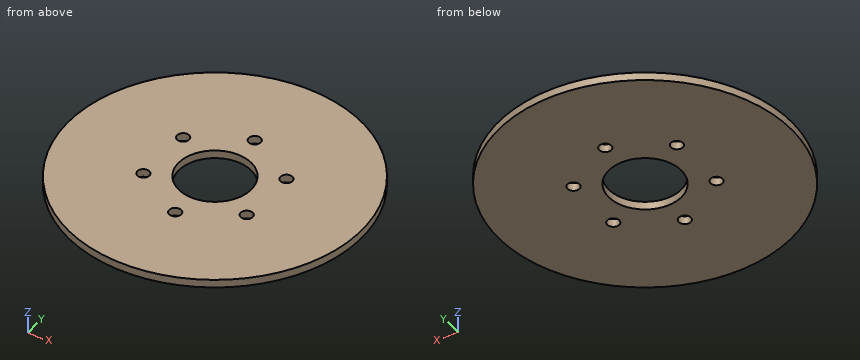
```python
from build123d import *

# Parameters (mm, degrees)
F0_R            = 57.15
F0_R_2          = 14.1605
F1_DEPTH        = 3.175
F2_R            = 2.3622
F3_DEPTH        = 3.176
F3_COPIES_COUNT = 6


# Not quite as in the source:
# - a pattern or mirror of a feature is missing from the dataset's text; its kind, count and spacing are read off the source's solid


with BuildPart() as f1:
    # F0 (on Top) → F1 (new body)
    with BuildSketch(Plane.XY):
        Circle(F0_R)
        Circle(F0_R_2, mode=Mode.SUBTRACT)
    extrude(amount=F1_DEPTH)

    # F2 (on face) → F3 (cut, through all)
    with BuildSketch(Plane.XY.offset(3.175)):
        with Locations((0, 23.8125)):
            Circle(F2_R)
    f3 = extrude(amount=-F3_DEPTH, mode=Mode.SUBTRACT)

    # F3_copies: F3 ×6 about axis
    f3_copies_axis = Axis((0, 0, 0), (0, 0, 1))
    for i in range(1, F3_COPIES_COUNT):
        add(f3.rotate(f3_copies_axis, i * 360 / F3_COPIES_COUNT), mode=Mode.SUBTRACT)


solid = f1.part
```
Read the model definition and answer for the solid it produces. Units are mm, in the model's axes. Coordinates: 2 decimals unless noted, no trailing zeros. Write each loop counter-clockwise with the first axis right and the second up, starting at its lowest first coordinate (ties: lowest second). Pieces come first, ordered by that corner, then holes. Notation, with made-up numbers: (-38.5, 35) - (1.5, 35) arc R18 ccw to (1.5, 68) - close; hole circle Ø11 at (-5, -4.75). An arc over 180 degrees is marked (long way). Answer as a JSON object with one key per item and string values. Group by question number.
1. A cutting plane is placed at A-A (x = 0). Give the number of separate pieces and of enclosed holes in the cut face, plus the area to 3 significant figures.
2. A cutting plane is placed at C-C (z = 1.55). Determine the outline of the cut face in (x, y).
3. Each of these flat-tipped pins is pushed along its axis until it touches: P1, Ø5.5, axis at x = -20.62, y = 11.91, coming from the +Z side (3 decimals); P2, Ø1, axis at x = 37.5, z = 1, coming from the -Y side; P3, Ø1.5, axis at x = -24.5, z = 0.5, coming from the -Y side; P4, Ø1.5, axis at y = -14.5, z = 1, coming from the +X side. Where does it stop, or does it pass through?
4. A cutting plane is placed at D-D (x = 49.5). Determine the outline of the cut face in (y, z) (3 decimals), plus the area to 3 significant figures.
5. Consider L1, parallel to X at y = 11.5, z = 2; L2, parallel to X at y = 10, z = 0.25; L3, parallel to Y at x = 1, z = 2.1. Determine where each line is inside the solid, lowest interval first. Write a range as [from, to].
Worked out:
{
 "1": {"separate pieces": "4", "enclosed holes": "0", "area": "243 mm²"},
 "2": {"outline": "circle Ø114.3 at (0, 0); hole circle Ø4.72 at (-20.62, -11.91); hole circle Ø4.72 at (-20.62, 11.91); hole circle Ø28.32 at (0, 0); hole circle Ø4.72 at (0, -23.81); hole circle Ø4.72 at (0, 23.81); hole circle Ø4.72 at (20.62, -11.91); hole circle Ø4.72 at (20.62, 11.91)"},
 "3": {"P1": "stops at z = 3.175", "P2": "stops at y = -43.56", "P3": "stops at y = -51.98", "P4": "stops at x = 55.47"},
 "4": {"outline": "(-28.563, 0) - (28.563, 0) - (28.563, 3.175) - (-28.563, 3.175) - close", "area": "181 mm²"},
 "5": {"L1": "x = [-55.98, -22.95], [-18.3, -8.26], [8.26, 18.3], [22.95, 55.98]", "L2": "x = [-56.27, -22.02], [-19.23, -10.03], [10.03, 19.23], [22.02, 56.27]", "L3": "y = [-57.14, -25.95], [-21.67, -14.13], [14.13, 21.67], [25.95, 57.14]"}
}
